The listing builds one solid part. Answer for the finished solid, in the listing's coordinates (mm). A direction names the side the tool comes from. Coordinates: 2 decimals unless noted, no trailing zeros. Order: outer loops, then holes, each group sorted by start corner. A loop starts at its lowest first (then second) coordinate and runs counter-clockwise, first axis right, second up.
from build123d import *

# Parameters (mm, degrees)
SKETCH3_W           = 43
SKETCH3_H           = 18.2
SKETCH3_R           = 2.1
BOSS_EXTRUDE5_DEPTH = 2
SKETCH1_R           = 3.75
BOSS_EXTRUDE1_DEPTH = 2
CHAMFER1_SIZE       = 1.5
SKETCH5_W           = 6
SKETCH5_H           = 9.25
BOSS_EXTRUDE4_DEPTH = 18.65
FILLET1_R           = 3


with BuildPart() as part:
    # Sketch3 → Boss-Extrude5 (new body)
    with BuildSketch(Plane(origin=(0, 0, 0), x_dir=(1, 0, 0), z_dir=(0, 1, 0))):
        with Locations((0, 9.1)):
            Rectangle(SKETCH3_W, SKETCH3_H)
        with Locations((-8, 8.1)):
            Circle(SKETCH3_R, mode=Mode.SUBTRACT)
        with Locations((8, 8.1)):
            Circle(SKETCH3_R, mode=Mode.SUBTRACT)
    extrude(amount=-BOSS_EXTRUDE5_DEPTH)

    # Sketch1 → Boss-Extrude1 (add)
    with BuildSketch(Plane.XY):
        Polygon((-43.85, -9.25), (-16.5, -9.25), (-16.5, -4), (16.5, -4), (16.5, -9.25), (43.85, -9.25), (43.85, 8.75), (16.5, 8.75), (16.5, 2), (-16.5, 2), (-16.5, 8.75), (-43.85, 8.75), align=None)
        with Locations((-27.85, -0.25)):
            Circle(SKETCH1_R, mode=Mode.SUBTRACT)
        with Locations((27.85, -0.25)):
            Circle(SKETCH1_R, mode=Mode.SUBTRACT)
    extrude(amount=BOSS_EXTRUDE1_DEPTH)

    # Chamfer1
    chamfer1_edges = [part.edges().sort_by_distance(p)[0] for p in [
        (0, -2, 0),
    ]]
    chamfer(chamfer1_edges, length=CHAMFER1_SIZE)

    # Sketch5 → Boss-Extrude4 (add)
    with BuildSketch(Plane(origin=(0, 0, 0), x_dir=(-1, 0, 0), z_dir=(0, 0, -1))):
        with Locations((40.85, -4.625)):
            Rectangle(SKETCH5_W, SKETCH5_H)
    boss_extrude4 = extrude(amount=BOSS_EXTRUDE4_DEPTH)

    # Mirror2: Boss-Extrude4 across plane
    add(boss_extrude4.mirror(Plane(origin=(0, 0, 0), x_dir=(0, 0, 1), z_dir=(1, 0, 0))))

    # Fillet1
    fillet1_edges = [part.edges().sort_by_distance(p)[0] for p in [
        (-43.85, 8.75, 1),
        (-43.85, -9.25, -8.325),
        (-16.5, -9.25, 1),
        (16.5, -9.25, 1),
        (43.85, -9.25, -8.325),
        (43.85, 8.75, 1),
        (16.5, 8.75, 1),
        (-16.5, 8.75, 1),
        (-43.85, 0, -9.325),
        (43.85, 0, -9.325),
    ]]
    fillet(fillet1_edges, radius=FILLET1_R)


solid = part.part
(1) Find section A-A on z = -8.1. Determine the outline of the cut face in (x, y).
(2) Find section B-B on z = -2.25. Determine the outline of the cut face in (x, y).
(3) A tool of negligible diameter and unlimited length cuts with its end or side. For faces 5 (the flat face through (-16.5, -5, 1)), 6 (the flat face through (-20, 2, 0)), 7 (the flat face through (-39, 0, -9)), 8 (the flat face through (-21.5, -1, -9)), 9 (the cylindrical face through (-17.36, 7.85, 1.01)), from which of +Z, -Z, +X, -X, +Y, -Y can it reach the whole face along a straight path? Write none if from no direction.
(4) Given pin 1 Ø2.5 at (x, z) = (39.5, -7.5) entering from +Y; pin 2 Ø8.5 at (x, y) = (27.85, -0.25) entering from -Z; pin 3 Ø1.8 at (y, z) = (-1, -12.5) entering from +X; pin 4 Ø4 at (y, z) = (-1.5, -7.5) entering from -X, each flat-ended and moving along its own axis, determine where each tip first touches the part or whether it passes through.
(5) Find section D-D on y = -7.5. Determine the outline of the cut face in (x, z).
(6) Find the intervals of material crossed by probe 1 along X at (y, z) = (-0.5, -8.1); probe 2 along X at (y, z) = (5.25, 0.25); probe 3 along X at (y, z) = (-1.5, -8.1), in increasing order.
(7) Find section C-C on x = 27.85. Determine the outline of the cut face in (y, z), then the cut area to 3 significant figures.
(8) The mould has two halves that part along Y. Classify faces 1 (the flat face through (21.5, -1, -9)), 2 (the cylindrical face through (17.36, -8.35, 1.01)), 3 (the cylindrical face through (-24.273, 0.876, 0.986)), 4 (the cylindrical face through (31.427, 0.876, 0.986)): pulls with the +Y half, pulls with the -Y half, needs draft (parallel to the pull), parting line crosses it, or undercut.
Resolved:
1. outline: (-43.85, -6.25) arc R3 ccw to (-40.85, -9.25) - (-37.85, -9.25) - (-37.85, 0) - (-40.85, 0) arc R3 ccw to (-43.85, -3) - close; (-21.5, -2) - (-10.1, -2) - (-10.1, 0) - (-21.5, 0) - close; (-5.9, -2) - (5.9, -2) - (5.9, 0) - (-5.9, 0) - close; (10.1, -2) - (21.5, -2) - (21.5, 0) - (10.1, 0) - close; (37.85, -9.25) - (40.85, -9.25) arc R3 ccw to (43.85, -6.25) - (43.85, -3) arc R3 ccw to (40.85, 0) - (37.85, 0) - close
2. outline: (-43.85, -6.25) arc R3 ccw to (-40.85, -9.25) - (-37.85, -9.25) - (-37.85, 0) - (-40.85, 0) arc R3 ccw to (-43.85, -3) - close; (-21.5, -2) - (21.5, -2) - (21.5, 0) - (-21.5, 0) - close; (37.85, -9.25) - (40.85, -9.25) arc R3 ccw to (43.85, -6.25) - (43.85, -3) arc R3 ccw to (40.85, 0) - (37.85, 0) - close
3. face 5: +Z, -Z, -Y
3. face 6: -Z
3. face 7: -Z, +X, -X, +Y
3. face 8: -Z, +Y, -Y
3. face 9: +Z, -Z, +Y
4. pin 1: stops at y = 0
4. pin 2: stops at z = 0
4. pin 3: stops at x = 43.64
4. pin 4: stops at x = -43.85
5. outline: (-43.58, -18.65) - (-37.85, -18.65) - (-37.85, 0) - (-16.77, 0) - (-16.77, 2) - (-43.58, 2) - close; (16.77, 0) - (37.85, 0) - (37.85, -18.65) - (43.58, -18.65) - (43.58, 2) - (16.77, 2) - close
6. probe 1: x = -42.51 to -37.85, -21.5 to -10.1, -5.9 to 5.9, 10.1 to 21.5, 37.85 to 42.51
6. probe 2: x = -43.85 to -16.5, 16.5 to 43.85
6. probe 3: x = -43.45 to -37.85, -21.5 to -10.1, -5.9 to 5.9, 10.1 to 21.5, 37.85 to 43.45
7. outline: (-9.25, 0) - (-4, 0) - (-4, 2) - (-9.25, 2) - close; (3.5, 0) - (8.75, 0) - (8.75, 2) - (3.5, 2) - close
7. area: 21.0 mm2
8. face 1: needs draft
8. face 2: pulls with the -Y half
8. face 3: undercut
8. face 4: undercut
